from build123d import *

# Parameters (mm, degrees)
F1_DEPTH = 28.575


# Not quite as in the source:
# - a feature names something its author has since deleted; it is built from what else it names


with BuildPart() as f1:
    # F0 (on Top) → F1 (new body)
    with BuildSketch(Plane.XY):
        with BuildLine():
            Line((304.8, 533.4), (-990.6, 533.4))
            Line((-990.6, 533.4), (-990.6, 0))
            Line((-990.6, 0), (-990.6, -533.4))
            Line((-990.6, -533.4), (304.8, -533.4))
            ThreePointArc((304.8, -533.4), (681.9707570849, -377.1707570849), (838.2, 0))
            ThreePointArc((838.2, 0), (681.9707570849, 377.1707570849), (304.8, 533.4))
        make_face()
        with BuildLine():
            ThreePointArc((-857.25, 0), (-901.7, -44.45), (-946.15, 0))
            ThreePointArc((-946.15, 0), (-901.7, 44.45), (-857.25, 0))
        make_face(mode=Mode.SUBTRACT)
    extrude(amount=F1_DEPTH)


solid = f1.part
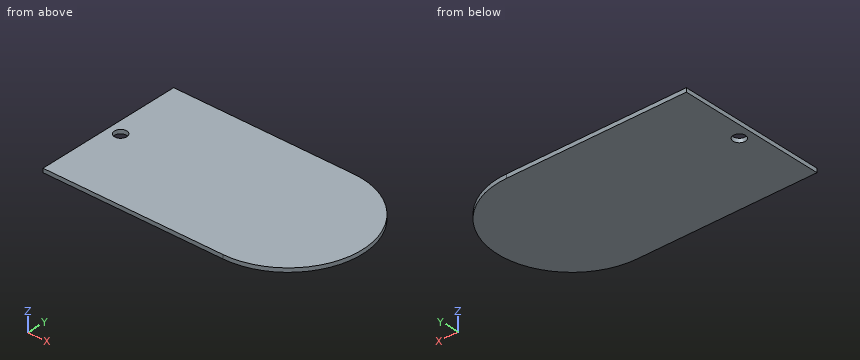
Geometry check sheet. Reference: the model listing, model coordinates, mm. Round coordinates to 2 decimals unless told otherwise and drop trailing zeros. Write each loop counter-clockwise with the first axis right and the second up, starting at its lowest first coordinate (ties: lowest second). Pieces come first, ordered by that corner, then holes. Notation, with made-up numbers: (5.25, 33) -> (39.25, 33) arc R35 ccw to (39.25, 72) -> close; hole circle Ø2 at (50.25, 21.25). An arc over 180 degrees is marked (long way). One line per item, written item: value. Start each with the question number.
(1) Cross-section at D-D, the plane y = -425. Record the cut outline in (x, z) (3 decimals).
(2) Cross-section at B-B, the plane z = 23.25. Record the cut outline in (x, y).
(3) Cross-section at A-A, the plane y = 0. Record the cut outline in (x, z) (3 decimals).
(4) Cross-section at C-C, the plane x = -901.7. Record the cut outline in (y, z) (3 decimals), and give its area (3 significant figures).
(5) Go/stop test with flat-tipped pins: pin 1 Ø8 at (x, z) = (528.5, 23) entering from +Y; pin 2 Ø1.5 at (y, z) = (-87.5, 19) entering from +X; pin 3 Ø3 at (x, z) = (626, 18.5) entering from +Y. Record where each tip stops, or that it passes through.
(6) Scan lines: line 1 (Y direction, x = -901.7, z = 21); line 2 (X direction, y = -24, z = 4); line 3 (X direction, y = 24.5, z = 14.75). Record each from-to range of solid material in increasing order. Write a range as [from, to].
Answer:
1. outline: (-990.6, 0) -> (627.121, 0) -> (627.121, 28.575) -> (-990.6, 28.575) -> close
2. outline: (-990.6, -533.4) -> (304.8, -533.4) arc R533.4 ccw to (304.8, 533.4) -> (-990.6, 533.4) -> close; hole circle Ø88.9 at (-901.7, 0)
3. outline: (-990.6, 0) -> (-946.15, 0) -> (-946.15, 28.575) -> (-990.6, 28.575) -> close; (-857.25, 0) -> (838.2, 0) -> (838.2, 28.575) -> (-857.25, 28.575) -> close
4. outline: (-533.4, 0) -> (-44.45, 0) -> (-44.45, 28.575) -> (-533.4, 28.575) -> close; (44.45, 0) -> (533.4, 0) -> (533.4, 28.575) -> (44.45, 28.575) -> close
4. area: 27,900 mm²
5. pin 1: y = 486.05
5. pin 2: x = 831.1
5. pin 3: y = 426.97
6. line 1: [-533.4, -44.45], [44.45, 533.4]
6. line 2: [-990.6, -939.11], [-864.29, 837.66]
6. line 3: [-990.6, -938.79], [-864.61, 837.64]
